from build123d import *

# Parameters (mm, degrees)
F0_R     = 2.5
F0_R_2   = 3.5
F0_W     = 40
F0_H     = 35
F0_R_3   = 1.5
F1_DEPTH = 5
F2_R     = 6
F2_R_2   = 6.5
F3_DEPTH = 5.001
F4_W     = 3
F4_H     = 7
F5_DEPTH = 5.001
F6_R     = 1.25
F7_DEPTH = 5.001
F8_R     = 5


with BuildPart() as f1:
    # F0 (on Top) → F1 (new body)
    with BuildSketch(Plane.XY):
        Polygon((35, -30), (35, 30), (-35, 30), (-35, -30), (-20, -30), (20, -30), align=None)
        with Locations((-25, -20.5)):
            Circle(F0_R, mode=Mode.SUBTRACT)
        with Locations((25, -20.5)):
            Circle(F0_R, mode=Mode.SUBTRACT)
        with Locations((-25, 20.5)):
            Circle(F0_R_2, mode=Mode.SUBTRACT)
        with Locations((25, 20.5)):
            Circle(F0_R_2, mode=Mode.SUBTRACT)
        with Locations((0, -47.5)):
            Rectangle(F0_W, F0_H)
        with Locations((-8.5, -57)):
            Circle(F0_R_3, mode=Mode.SUBTRACT)
        with Locations((8.5, -57)):
            Circle(F0_R_3, mode=Mode.SUBTRACT)
        with Locations((0, -45)):
            Circle(F0_R_3, mode=Mode.SUBTRACT)
    extrude(amount=F1_DEPTH)

    # F2 (on face) → F3 (cut, through all)
    with BuildSketch(Plane.XY.offset(5)):
        with Locations((-9, -48)):
            Circle(F2_R)
        with Locations((9, -48)):
            Circle(F2_R)
        with Locations((0, -31.5)):
            Circle(F2_R_2)
    extrude(amount=-F3_DEPTH, mode=Mode.SUBTRACT)

    # F4 (on face) → F5 (cut, through all)
    with BuildSketch(Plane.XY.offset(5)):
        with Locations((28.5, 0.5)):
            Rectangle(F4_W, F4_H)
        with Locations((-28.5, 0.5)):
            Rectangle(F4_W, F4_H)
    extrude(amount=-F5_DEPTH, mode=Mode.SUBTRACT)

    # F6 (on face) → F7 (cut, through all)
    with BuildSketch(Plane.XY.offset(5)):
        with Locations((-30, -6.5)):
            Circle(F6_R)
        with Locations((-30, -12.5)):
            Circle(F6_R)
    extrude(amount=-F7_DEPTH, mode=Mode.SUBTRACT)

    # F8
    f8_edges = [f1.edges().sort_by_distance(p)[0] for p in [
        (-20, -30, 2.5),
        (-20, -65, 2.5),
        (20, -65, 2.5),
        (20, -30, 2.5),
        (35, -30, 2.5),
        (35, 30, 2.5),
        (-35, 30, 2.5),
        (-35, -30, 2.5),
    ]]
    fillet(f8_edges, radius=F8_R)


solid = f1.part
Check sheet for the modelled part. Datum: model origin and axes. Units: mm. A direction names the side the tool comes from. Give positions to 0.01 mm unless a question says otherwise; leave off trailing zeros. Loops run counter-clockwise (first coordinate to the right, second up) from the corner with the lowest first, then second, coordinate; pieces in that order, holes last. Notation, with made-up numbers: M -18.75,89 L -0.75,89 A27 cw -0.75,126 Z; hole C 13,41 d11. An arc over 180 degrees is marked long. Return JSON: item names as keys, results as strings. Group by question number.
1. Cross-section at D-D on z = 1.95. State how many separate pieces and enclosed holes the cut face has, plus the area to 3 significant figures.
2. Tool access check on faces 1 (the flat face through (-29, 4, 3)), 2 (the cylindrical face through (22, -31, 3)). Record the directions out of +Z, -Z, +X, -X, +Y, -Y that give a thin tool (end or side, any length) a straight path to the whole face; none if there is none.
3. Cross-section at C-C on y = -45. Record the boundary of the cut face in (x, z), plus the area to 3 significant figures.
4. Mould release check, pull along Y, two halves, no side actions. Record for faces 3 (the flat face through (27, 0, 3)), 4 (the flat face through (0, -65, 2)), 5 (the flat face through (20, -48, 2)): released by +Y, released by -Y, zero draft, split by the parting line, or undercut.
5. Cross-section at A-A on y = -57. Record the boundary of the cut face in (x, z).
6. Thickness scan on L1, parallel to X at y = -2.5, z = 4; L2, parallel to Y at x = 0, z = 1.9; L3, parallel to Y at x = -3.5, z = 3.95. Record the ranges inside material, lowest first.
7. Cross-section at B-B on x = 5. Record the boundary of the cut face in (y, z).
8. Go/stop test with flat-tipped pins: pin 1 (2 mm diameter, centred on x = -17, z = 3, fed in from -Y); pin 2 (1.5 mm diameter, centred on y = -52, z = 1.5, fed in from -X); pin 3 (1 mm diameter, centred on y = -48, z = 2.5, fed in from +X). Record where each tip stops, or that it passes through.
Return value:
{
 "1": {"separate pieces": "1", "enclosed holes": "14", "area": "5,030 mm^2"},
 "2": {"face 1": "+Z, -Z", "face 2": "+Z, -Z, +X, -Y"},
 "3": {"outline": "M -20,0 L -14.2,0 L -14.2,5 L -20,5 Z; M -3.8,0 L -1.5,0 L -1.5,5 L -3.8,5 Z; M 1.5,0 L 3.8,0 L 3.8,5 L 1.5,5 Z; M 14.2,0 L 20,0 L 20,5 L 14.2,5 Z", "area": "81.1 mm^2"},
 "4": {"face 3": "undercut", "face 4": "released by -Y", "face 5": "zero draft"},
 "5": {"outline": "M -20,0 L -10,0 L -10,5 L -20,5 Z; M -7,0 L 7,0 L 7,5 L -7,5 Z; M 10,0 L 20,0 L 20,5 L 10,5 Z"},
 "6": {"L1": "-35 to -30, -27 to 27, 30 to 35", "L2": "-65 to -46.5, -43.5 to -38, -25 to 30", "L3": "-65 to -50.4, -45.6 to -36.98, -26.02 to 30"},
 "7": {"outline": "M -65,0 L -52.47,0 L -52.47,5 L -65,5 Z; M -43.53,0 L -35.65,0 L -35.65,5 L -43.53,5 Z; M -27.35,0 L 30,0 L 30,5 L -27.35,5 Z"},
 "8": {"pin 1": "y = -64.9", "pin 2": "x = -20", "pin 3": "x = 20"}
}
